from build123d import *

# Parameters (mm, degrees)
SKETCH1_W           = 60
SKETCH1_H           = 50
BOSS_EXTRUDE1_DEPTH = 5
CHAMFER1_SIZE       = 2
SKETCH2_R           = 1.55
CUT_EXTRUDE1_DEPTH  = 2
CUT_EXTRUDE2_REACH  = 7
SKETCH3_R           = 1.55


with BuildPart() as part:
    # Sketch1 → Boss-Extrude1 (new body)
    with BuildSketch(Plane(origin=(0, 0, 0), x_dir=(1, 0, 0), z_dir=(0, 1, 0))):
        with Locations((30, 25)):
            Rectangle(SKETCH1_W, SKETCH1_H)
    extrude(amount=BOSS_EXTRUDE1_DEPTH)

    # Chamfer1
    chamfer1_edges = [part.edges().sort_by_distance(p)[0] for p in [
        (0, 2.5, -50),
        (60, 2.5, -50),
        (60, 2.5, 0),
        (0, 2.5, 0),
    ]]
    chamfer(chamfer1_edges, length=CHAMFER1_SIZE)

    # Sketch2 → Cut-Extrude1 (cut)
    with BuildSketch(Plane(origin=(0, 5, 0), x_dir=(1, 0, 0), z_dir=(0, 1, 0))):
        with Locations((55.5, 4.5)):
            Circle(SKETCH2_R)
        with Locations((4.5, 4.5)):
            Circle(SKETCH2_R)
        with Locations((4.5, 45.5)):
            Circle(SKETCH2_R)
        with Locations((55.5, 45.5)):
            Circle(SKETCH2_R)
    extrude(amount=-CUT_EXTRUDE1_DEPTH, mode=Mode.SUBTRACT)

    # Sketch3 → Cut-Extrude2 (cut, up to next)
    with BuildSketch(Plane(origin=(0, 5, 0), x_dir=(1, 0, 0), z_dir=(0, 1, 0)), mode=Mode.PRIVATE) as cut_extrude2_sk1:
        with Locations((42, 29.446052378)):
            Circle(SKETCH3_R)
    cut_extrude2_tool1 = extrude(cut_extrude2_sk1.sketch, amount=-CUT_EXTRUDE2_REACH, mode=Mode.PRIVATE) & part.part
    add(cut_extrude2_tool1.solids().sort_by_distance((42, 5, -29.446052))[0], mode=Mode.SUBTRACT)
    # Sketch3 → Cut-Extrude2 (cut, up to next)
    with BuildSketch(Plane(origin=(0, 5, 0), x_dir=(1, 0, 0), z_dir=(0, 1, 0)), mode=Mode.PRIVATE) as cut_extrude2_sk2:
        with Locations((29, 29.446052378)):
            Circle(SKETCH3_R)
    cut_extrude2_tool2 = extrude(cut_extrude2_sk2.sketch, amount=-CUT_EXTRUDE2_REACH, mode=Mode.PRIVATE) & part.part
    add(cut_extrude2_tool2.solids().sort_by_distance((29, 5, -29.446052))[0], mode=Mode.SUBTRACT)
    # Sketch3 → Cut-Extrude2 (cut, up to next)
    with BuildSketch(Plane(origin=(0, 5, 0), x_dir=(1, 0, 0), z_dir=(0, 1, 0)), mode=Mode.PRIVATE) as cut_extrude2_sk3:
        with Locations((42, 18.509029021)):
            Circle(SKETCH3_R)
    cut_extrude2_tool3 = extrude(cut_extrude2_sk3.sketch, amount=-CUT_EXTRUDE2_REACH, mode=Mode.PRIVATE) & part.part
    add(cut_extrude2_tool3.solids().sort_by_distance((42, 5, -18.509029))[0], mode=Mode.SUBTRACT)
    # Sketch3 → Cut-Extrude2 (cut, up to next)
    with BuildSketch(Plane(origin=(0, 5, 0), x_dir=(1, 0, 0), z_dir=(0, 1, 0)), mode=Mode.PRIVATE) as cut_extrude2_sk4:
        with Locations((29, 18.509029021)):
            Circle(SKETCH3_R)
    cut_extrude2_tool4 = extrude(cut_extrude2_sk4.sketch, amount=-CUT_EXTRUDE2_REACH, mode=Mode.PRIVATE) & part.part
    add(cut_extrude2_tool4.solids().sort_by_distance((29, 5, -18.509029))[0], mode=Mode.SUBTRACT)


solid = part.part
Design review of the part built by this model. Coordinates are the model's own, in mm. A direction names the side the tool comes from. Coordinates: 2 decimals unless noted, no trailing zeros. Loops run counter-clockwise (first coordinate to the right, second up) from the corner with the lowest first, then second, coordinate; pieces in that order, holes last.
Item 1: Add section C-C (x = 4.5). Write out the cut boundary in (y, z), and give its area (3 significant figures).
Completed:
outline: (0, -50) - (5, -50) - (5, -47.05) - (3, -47.05) - (3, -43.95) - (5, -43.95) - (5, -6.05) - (3, -6.05) - (3, -2.95) - (5, -2.95) - (5, 0) - (0, 0) - close
area: 238 mm2
Item 2: Add section A-A (x = 42). Write out the cut boundary in (y, z).
Completed:
outline: (0, -50) - (5, -50) - (5, -31) - (0, -31) - close; (0, -27.9) - (5, -27.9) - (5, -20.06) - (0, -20.06) - close; (0, -16.96) - (5, -16.96) - (5, 0) - (0, 0) - close
Item 3: Draft analysis for pull direction X (two halves, no side actions). For faces 3 (the cylindrical face through (4.164, 4.014, -43.987)), 4 (the flat face through (30, 2, -50)), 5 (the flat face through (1, 2, -49)), 6 (the cylindrical face through (43.43, 2.54, -28.85)), state which applies: pulls with the +X half, pulls with the -X half, needs draft (parallel to the pull), parting line crosses it, or undercut.
Completed:
face 3: undercut
face 4: needs draft
face 5: pulls with the -X half
face 6: undercut
Item 4: For faces 1 (the flat face through (30, 0, -25)), 2 (the cylindrical face through (56.978, 4.014, -4.966)), list the 3-axis set-ups (+Z, -Z, +X, -X, +Y, -Y) from which the entire face can be reached by the end or side of a thin tool; tool diameter is ignored.
Completed:
face 1: +Z, -Z, +X, -X, -Y
face 2: +Y
Item 5: Clearance check with flat-ended pins moving along their axes: pin 1 (1.5 mm diameter, centred on x = 5, z = -45.5, fed in from +Y); pin 2 (1.9 mm diameter, centred on x = 29, z = -18.51, fed in from +Y). State where each tip first meets the part, or that it passes through.
Completed:
pin 1: stops at y = 3
pin 2: passes through
Item 6: Add section B-B (z = -45.5). Write out the cut boundary in (x, y), and give its area (3 significant figures).
Completed:
outline: (0, 0) - (60, 0) - (60, 5) - (57.05, 5) - (57.05, 3) - (53.95, 3) - (53.95, 5) - (6.05, 5) - (6.05, 3) - (2.95, 3) - (2.95, 5) - (0, 5) - close
area: 288 mm2
Item 7: Wall thickness on L1, parallel to X at y = 3.95, z = -4.5; L2, parallel to Z at x = 29, y = 2.4; L3, parallel to Z at x = 4.5, y = 4.05: over which ranges is each line inside the solid? List them lowest first.
Completed:
L1: x = 0 to 2.95, 6.05 to 53.95, 57.05 to 60
L2: z = -50 to -31, -27.9 to -20.06, -16.96 to 0
L3: z = -50 to -47.05, -43.95 to -6.05, -2.95 to 0
